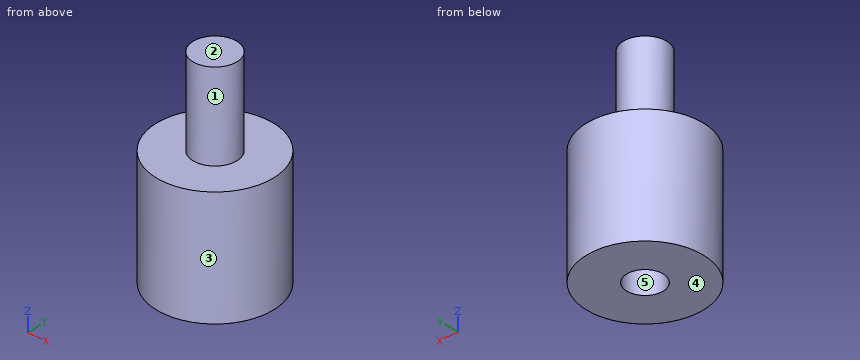
Autodesk Inventor part; units mm, degrees
ref_plane "YZ Plane" through (0, 0, 0) normal (1, 0, 0) x (0, 1, 0)
ref_plane "XZ Plane" through (0, 0, 0) normal (0, 1, 0) x (-1, 0, 0)
ref_plane "XY Plane" through (0, 0, 0) normal (0, 0, 1) x (1, 0, 0)
sketch "スケッチ1" plane through (0, 0, 0) normal (0, 0, 1) x (1, 0, 0)
  circle A0 centre (0, 0) radius 4
  circle A1 centre (0, 0) radius 1.5
  dimension "d0" = 8
  dimension "d1" = 3
extrude "押し出し1" add sketch "スケッチ1" along normal blind 6 contours A1
extrude "押し出し2" add sketch "スケッチ1" against normal blind 8 contours A0 | A1
sketch "スケッチ2" plane through (0, 0, -8) normal (0, 0, -1) x (-1, 0, 0)
  circle A0 centre (0, 0) radius 4
hole "穴1" at (0, 0, -8) direction (0, 0, 1) diameter 2.5 depth 3 tip angle 118
properties part number "防振ゴム雄ねじ雌ねじスペーサー"
The model under review builds one solid part; all positions refer to its coordinate system, in mm. Face numbers are marked on the shaded views. A direction names the side the tool comes from. Round coordinates to 2 decimals unless told otherwise and drop trailing zeros. Loops run counter-clockwise (first coordinate to the right, second up) from the corner with the lowest first, then second, coordinate; pieces in that order, holes last. Notation, with made-up numbers: (28.25, 48) - (65.25, 48) arc R16 cw to (65.25, 74) - close; hole circle Ø6 at (-27, 25). An arc over 180 degrees is marked (long way). Use a Markdown table: item, result. Add a question column.
Q1. The part is to be moulded in two halves that separate along Y. For the marked faces 3, 4 and 5, say which applies: pulls with the +Y half, pulls with the -Y half, needs draft (parallel to the pull), parting line crosses it, or undercut.
Q2. Add section C-C (x = -2.5). State the section outline as (y, z) points.
Q3. Add section B-B (z = -3). State the section outline as (x, y) points, plus the area to 3 significant figures.
Q4. Add section D-D (y = 3). State the section outline as (x, z) points.
Q5. Add section A-A (z = -7). State the section outline as (x, y) points.
Q6. Machinability: for the marked faces 1 and 2, which of the approach directions +Z, -Z, +X, -X, +Y, -Y give a long, thin tool a straight path to every point of the face, cutting with its end or side? Answer none if there is none.
Q7. For probe 1 along Y at (x, z) = (0, -6.9); probe 2 along Z at (x, y) = (-2.5, 1.25); probe 3 along X at (y, z) = (-3.25, -4), list the stretches that pass through material, from the lowest coordinate up.
Q8. Insertion check: pin 1 Ø1.5 at (y, z) = (-3, -2.5) entering from +X; pin 2 Ø2 at (y, z) = (2, 1.5) entering from +X; pin 3 Ø1 at (x, z) = (0, 1) entering from +Y; pin 4 Ø2.5 at (x, y) = (-1.5, 0.5) entering from +Z. Each pin has a flat end and moves straight along its axis. Give the tip position at first contact, or say it passes through.
Worked answers:
| question | item | result |
|---|---|---|
| 1 | face 3 | parting line crosses it |
| 1 | face 4 | needs draft |
| 1 | face 5 | undercut |
| 2 | outline | (-3.12, -8) - (3.12, -8) - (3.12, 0) - (-3.12, 0) - close |
| 3 | outline | circle Ø8 at (0, 0) |
| 3 | area | 50.3 mm² |
| 4 | outline | (-2.65, -8) - (2.65, -8) - (2.65, 0) - (-2.65, 0) - close |
| 5 | outline | circle Ø8 at (0, 0); hole circle Ø2.5 at (0, 0) |
| 6 | face 1 | +Z |
| 6 | face 2 | +Z, +X, -X, +Y, -Y |
| 7 | probe 1 | -4 to -1.25, 1.25 to 4 |
| 7 | probe 2 | -8 to 0 |
| 7 | probe 3 | -2.33 to 2.33 |
| 8 | pin 1 | x = 3.31 |
| 8 | pin 2 | x = 1.12 |
| 8 | pin 3 | y = 1.5 |
| 8 | pin 4 | z = 6 |
